from build123d import *

# Parameters (mm, degrees)
SKETCH_1_R      = 1.75
EXTRUDE_1_DEPTH = 8.5


with BuildPart() as part:
    # 草图1 → 凸台-拉伸1 (new body)
    with BuildSketch(Plane(origin=(0, 0, 0), x_dir=(1, 0, 0), z_dir=(0, 1, 0))):
        with BuildLine():
            Line((-5, 0), (-5, 24))
            Line((-5, 24), (-1.652561305, 30.147735696))
            ThreePointArc((-1.652561305, 30.147735696), (10.212693953, 40.487182849), (13.939150793, 55.777767179))
            Line((13.939150793, 55.777767179), (17.049795585, 61.490619233))
            ThreePointArc((17.049795585, 61.490619233), (17.188178873, 47.06817383), (10.58000386, 34.247951355))
            Line((10.58000386, 34.247951355), (5, 24))
            Line((5, 24), (5, 0))
            ThreePointArc((5, 0), (0, -5), (-5, 0))
        make_face()
        with Locations(Location((0, 0, 0), (0, 0, 270))):
            Circle(SKETCH_1_R, mode=Mode.SUBTRACT)
        with Locations(Location((0, 22, 0), (0, 0, 270))):
            Circle(SKETCH_1_R, mode=Mode.SUBTRACT)
    extrude(amount=EXTRUDE_1_DEPTH)


solid = part.part
Source: CAD feature listing. Evaluate the final solid. Frame: model axes, mm. A direction names the side the tool comes from. Give positions to 0.01 mm unless a question says otherwise; leave off trailing zeros. Write each loop counter-clockwise with the first axis right and the second up, starting at its lowest first coordinate (ties: lowest second). Pieces come first, ordered by that corner, then holes. Notation, with made-up numbers: (67, 42) -> (87, 42) arc R28 ccw to (87, 75) -> close; hole circle Ø11 at (55.5, 77). An arc over 180 degrees is marked (long way). Return JSON: item names as keys, results as strings. Group by question number.
1. Pin query (flat end, axial travel): pin 1 Ø4.5 at (x, z) = (0, -22) entering from +Y; pin 2 Ø4 at (y, z) = (3, -29) entering from +X; pin 3 Ø1 at (x, y) = (4.5, 3.5) entering from +Z. Return the tip coordinate at first contact, or that it passes through.
2. Access query for faces 1 (the face through (0.08, 4.19, -23.75)), 2 (the face through (5, 4, -12)). Directions: +Z, -Z, +X, -X, +Y, -Y. A direction counts if a zero-diameter tool reaches every point of the face in a straight line with its end or side. Return the directions, or none.
3. Section D-D, the plane z = -1. Output: boundary loops of the cut face in (x, y).
4. Material intervals for line 1 (X direction, y = 5, z = -20); line 2 (X direction, y = 2, z = -21.5); line 3 (X direction, y = 0.75, z = -38.5), sorted ascending. Write a range as from..to.
5. Mould query, pull axis X, two halves, no side actions, for faces 3 (the face through (-1.71, 4.19, -0.38)), 4 (the face through (3, 0, -23)), 5 (the face through (-3.35, 4.19, -27.03)). Classes: +X half, -X half, draft (parallel to the pull), parting line (faces both ways), or undercut.
6. Section C-C, the plane y = 3. Output: boundary loops of the cut face in (x, z), then the cut area to 3 significant figures.
7. Section B-B, the plane x = 0. Output: boundary loops of the cut face in (y, z), then the cut area to 3 significant figures.
8. Section A-A, the plane z = -22. Output: boundary loops of the cut face in (x, y), then the cut area to 4 significant figures.
Determined:
{
 "1": {"pin 1": "stops at y = 8.5", "pin 2": "stops at x = 8.81", "pin 3": "stops at z = 3"},
 "2": {"face 1": "+Y, -Y", "face 2": "+Z, +X, +Y, -Y"},
 "3": {"outline": "(-5, 0) -> (-1.44, 0) -> (-1.44, 8.5) -> (-5, 8.5) -> close; (1.44, 0) -> (5, 0) -> (5, 8.5) -> (1.44, 8.5) -> close"},
 "4": {"line 1": "x = -5..5", "line 2": "x = -5..-1.68, 1.68..5", "line 3": "x = 8.87..13.69"},
 "5": {"face 3": "undercut", "face 4": "draft", "face 5": "-X half"},
 "6": {"outline": "(-5, -24) -> (-1.65, -30.15) arc R26 cw to (13.94, -55.78) -> (17.05, -61.49) arc R30 ccw to (10.58, -34.25) -> (5, -24) -> (5, 0) arc R5 ccw to (-5, 0) -> close; hole circle Ø3.5 at (0, -22); hole circle Ø3.5 at (0, 0)", "area": "459 mm2"},
 "7": {"outline": "(0, -30.93) -> (8.5, -30.93) -> (8.5, -23.75) -> (0, -23.75) -> close; (0, -20.25) -> (8.5, -20.25) -> (8.5, -1.75) -> (0, -1.75) -> close; (0, 1.75) -> (8.5, 1.75) -> (8.5, 5) -> (0, 5) -> close", "area": "246 mm2"},
 "8": {"outline": "(-5, 0) -> (-1.75, 0) -> (-1.75, 8.5) -> (-5, 8.5) -> close; (1.75, 0) -> (5, 0) -> (5, 8.5) -> (1.75, 8.5) -> close", "area": "55.25 mm2"}
}
